For this review, take the finished solid that the model builds, in its own axes (mm). Face numbers are marked on the shaded views. A direction names the side the tool comes from. Coordinates: 2 decimals unless noted, no trailing zeros. Loops run counter-clockwise (first coordinate to the right, second up) from the corner with the lowest first, then second, coordinate; pieces in that order, holes last. Notation, with made-up numbers: (62.5, 86) - (90.5, 86) arc R18 ccw to (90.5, 93) - close; hole circle Ø7 at (-23, -21). An arc over 180 degrees is marked (long way). Answer as a JSON object with one key per item and string values. Group by question number.
Item 1: Clearance check with flat-ended pins moving along their axes: pin 1 (5 mm diameter, centred on x = 0, z = 37, fed in from +Y) (3 decimals); pin 2 (5 mm diameter, centred on x = 1, y = 0.5, fed in from -Z); pin 3 (3 mm diameter, centred on y = -0.5, z = 65, fed in from -X) (3 decimals). State where each tip first meets the part, or that it passes through.
Item 2: We need section A-A (z = 63.5). Give the boundary of the cut face in (x, y) (3 decimals), then the cut area to 3 significant figures.
Item 3: Tool access review of the marked faces 1 and 2: name each direction out of +Z, -Z, +X, -X, +Y, -Y from which nothing blocks a thin tool from reaching the whole face with its end or side.
Item 4: To check wall thickness, follow line 1 (Z direction, x = 0.5, y = -1.25) (3 decimals); line 2 (Z direction, x = 0.75, y = 3.75); line 3 (Y direction, x = 0.25, z = 69.5). State the ranges of each line that lie inside material, in increasing order.
Autodesk Inventor part; units mm, degrees
ref_plane "YZ Plane" through (0, 0, 0) normal (1, 0, 0) x (0, 1, 0)
ref_plane "XZ Plane" through (0, 0, 0) normal (0, 1, 0) x (-1, 0, 0)
ref_plane "XY Plane" through (0, 0, 0) normal (0, 0, 1) x (1, 0, 0)
sketch "Sketch1" plane through (0, 0, 0) normal (0, 0, 1) x (1, 0, 0)
  circle A0 centre (0, 0) radius 3.175
  dimension "d0" = 6.35
extrude "Extrusion1" add sketch "Sketch1" along normal blind 76.2
sketch "Sketch2" plane through (0, 0, 0) normal (0, 0, -1) x (-1, 0, 0)
  circle A0 centre (0, 0) radius 3.175
  circle A1 centre (0, 0) radius 4.7625
  dimension "d3" = 9.525
extrude "Extrusion2" add sketch "Sketch2" along normal blind 6.35 contours A0 | A1
sketch "Sketch3" plane through (0, 0, -6.35) normal (0, 0, -1) x (-1, 0, 0)
  circle A0 centre (0, 0) radius 4.7625
  line L0 (-1.3748, 2.3812) -> (1.3748, 2.3813)
  line L1 (1.3748, 2.3813) -> (2.7496, 0)
  line L2 (2.7496, 0) -> (1.3748, -2.3812)
  line L3 (1.3748, -2.3812) -> (-1.3748, -2.3812)
  line L4 (-1.3748, -2.3812) -> (-2.7496, 0)
  line L5 (-2.7496, 0) -> (-1.3748, 2.3812)
  dimension "d6" = 4.7625
extrude "Extrusion3" cut sketch "Sketch3" against normal blind 3.175 contours L0 L1 L2 L3 L4 L5
chamfer "Chamfer1" distance 0.508 angle 45 3 edges at (-3.175, 0, 76.2) (4.7625, 0, 0) (4.7625, 0, -6.35)
thread "Thread1"
properties part number "14-20 x750" material "Steel"
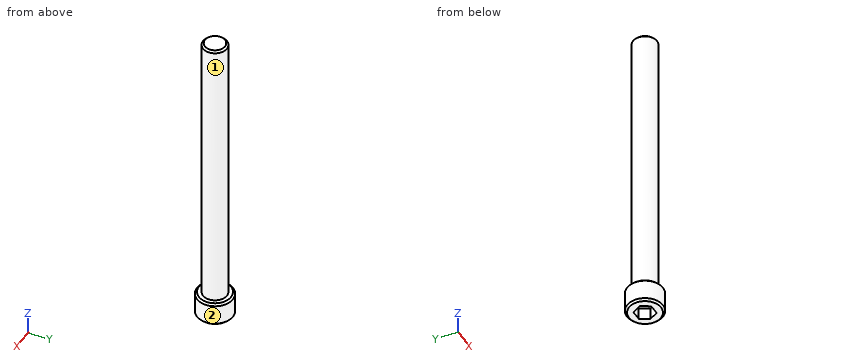
Check sheet entries:
{
 "1": {"pin 1": "stops at y = 3.175", "pin 2": "stops at z = -6.35", "pin 3": "stops at x = -3.175"},
 "2": {"outline": "circle Ø6.35 at (0, 0)", "area": "31.7 mm2"},
 "3": {"face 1": "+Z", "face 2": "+Z, -Z"},
 "4": {"line 1": "z = -3.175 to 76.2", "line 2": "z = -6.35 to 0", "line 3": "y = -3.17 to 3.17"}
}
